from build123d import *

# Parameters (mm, degrees)
BOSS_EXTRU_1_DEPTH      = 50
ESQUISSE2_R             = 8
ENL_V_MAT_EXTRU_1_DEPTH = 42.5
BOSS_EXTRU_3_DEPTH      = 2
BOSS_EXTRU_4_DEPTH      = 8
BOSS_EXTRU_5_DEPTH      = 8.222835
ESQUISSE8_R             = 1.65
ESQUISSE8_R_2           = 3
BOSS_EXTRU_6_DEPTH      = 6.507031
ESQUISSE9_R             = 10.5
ENL_V_MAT_EXTRU_2_DEPTH = 5.007031


with BuildPart() as part:
    # Esquisse1 → Boss.-Extru.1 (new body)
    with BuildSketch(Plane(origin=(0, 0, 0), x_dir=(1, 0, 0), z_dir=(0, 1, 0))):
        with BuildLine():
            ThreePointArc((-34.715340416, 22.739726027), (-41.5, 0), (-34.715340416, -22.739726027))
            ThreePointArc((-34.715340416, -22.739726027), (-31.254191835, -23.461148581), (-30.532769282, -20))
            ThreePointArc((-30.532769282, -20), (-36.5, 0), (-30.532769282, 20))
            ThreePointArc((-30.532769282, 20), (-31.254191835, 23.461148581), (-34.715340416, 22.739726027))
        make_face()
    extrude(amount=BOSS_EXTRU_1_DEPTH)

    # Esquisse2 → Enlèv. mat.-Extru.1 (cut, through all)
    with BuildSketch(Plane(origin=(0, 0, 0), x_dir=(0, 0, -1), z_dir=(1, 0, 0))):
        with Locations((0, 35)):
            Circle(ESQUISSE2_R)
    extrude(amount=-ENL_V_MAT_EXTRU_1_DEPTH, mode=Mode.SUBTRACT)



with BuildPart() as body_2:
    # Esquisse4 → Boss.-Extru.3 (new body)
    with BuildSketch(Plane.ZY.offset(56.5)):
        with BuildLine():
            Line((-2.6, 35), (-2.6, 45))
            Line((-2.6, 45), (-10, 45))
            Line((-10, 45), (-10, 25))
            Line((-10, 25), (10, 25))
            Line((10, 25), (10, 45))
            Line((10, 45), (2.6, 45))
            Line((2.6, 45), (2.6, 35))
            ThreePointArc((2.6, 35), (0, 32.4), (-2.6, 35))
        make_face()
    extrude(amount=BOSS_EXTRU_3_DEPTH)

    # Esquisse6 → Boss.-Extru.4 (add)
    with BuildSketch(Plane.ZY.offset(56.5)):
        Polygon((6.05, 31.507030871), (0, 28.014061743), (-6.05, 31.507030871), (-10, 31.507030871), (-10, 25), (10, 25), (10, 31.507030871), align=None)
    extrude(amount=-BOSS_EXTRU_4_DEPTH)


with BuildPart() as part_1:
    add(part.part)

    add(body_2.part)  # Boss.-Extru.5 merges body 2
    # Esquisse7 → Boss.-Extru.5 (add)
    with BuildSketch(Plane(origin=(-48.5, 0, 0), x_dir=(0, 0, -1), z_dir=(1, 0, 0))):
        with BuildLine():
            Line((10, 31.507030871), (7.197163793, 31.507030871))
            ThreePointArc((7.197163793, 31.507030871), (0, 27), (-7.197163793, 31.507030871))
            Line((-7.197163793, 31.507030871), (-10, 31.507030871))
            Line((-10, 31.507030871), (-10, 25))
            Line((-10, 25), (10, 25))
            Line((10, 25), (10, 31.507030871))
        make_face()
    extrude(amount=BOSS_EXTRU_5_DEPTH)

    # Esquisse8 → Boss.-Extru.6 (add)
    with BuildSketch(Plane.XZ.offset(-25)):
        with BuildLine():
            Line((-54.388582373, 10), (-44.388582373, 10))
            add(Edge.make_bspline(
                [(-82.50013532, 49), (-49.000452969, 40.897437534), (-44.388582373, 10)],
                knots=[0, 0, 0, 1, 1, 1], degree=2))
            ThreePointArc((-82.50013532, 49), (-107.50013532, 44), (-82.50013532, 39))
            add(Edge.make_bspline(
                [(-82.50013532, 39), (-57.708994437, 32.301835207), (-54.388582373, 10)],
                knots=[0, 0, 0, 1, 1, 1], degree=2))
        make_face()
        with Locations((-87.50013532, 44)):
            Circle(ESQUISSE8_R, mode=Mode.SUBTRACT)
        with Locations((-94.50013532, 37)):
            Circle(ESQUISSE8_R, mode=Mode.SUBTRACT)
        with Locations((-101.50013532, 44)):
            Circle(ESQUISSE8_R, mode=Mode.SUBTRACT)
        with Locations((-94.50013532, 51)):
            Circle(ESQUISSE8_R, mode=Mode.SUBTRACT)
        with Locations((-94.50013532, 44)):
            Circle(ESQUISSE8_R_2, mode=Mode.SUBTRACT)
    extrude(amount=-BOSS_EXTRU_6_DEPTH)

    # Esquisse9 → Enlèv. mat.-Extru.2 (cut)
    with BuildSketch(Plane.XZ.offset(-25)):
        with Locations((-94.50013532, 44)):
            Circle(ESQUISSE9_R)
    extrude(amount=-ENL_V_MAT_EXTRU_2_DEPTH, mode=Mode.SUBTRACT)


solid = part_1.part
Geometry check sheet. Reference: the model listing, model coordinates, mm. A direction names the side the tool comes from. Give positions to 0.01 mm unless a question says otherwise; leave off trailing zeros. Order: outer loops, then holes, each group sorted by start corner. A loop starts at its lowest first (then second) coordinate and runs counter-clockwise, first axis right, second up. Notation, with made-up numbers: (84.25, 85) - (100.25, 85) arc R30 ccw to (100.25, 118) - close; hole circle Ø6 at (29, 34.25). An arc over 180 degrees is marked (long way). Answer as a JSON object with one key per item and string values.
(1) Cross-section at B-B (z = 51). Record the cut outline in (x, y), then the cut area to 3 significant figures.
Report:
{"outline": "(-105.45, 25) - (-102.33, 25) - (-102.33, 30.01) - (-96.15, 30.01) - (-96.15, 31.51) - (-105.45, 31.51) - close; (-92.85, 30.01) - (-86.67, 30.01) - (-86.67, 25) - (-83.55, 25) - (-83.55, 31.51) - (-92.85, 31.51) - close", "area": "59.2 mm^2"}
(2) Cross-section at C-C (x = -43). Record the cut outline in (y, z), then the cut area to 3 significant figures.
Report:
{"outline": "(25, -10) - (31.51, -10) - (31.51, -7.2) arc R8 cw to (31.51, 7.2) - (31.51, 10) - (25, 10) - close", "area": "83.7 mm^2"}
(3) Material ranges on line 1 (Y direction, x = -39.6, z = 0); line 2 (Z direction, x = -94.5, y = 28.5); line 3 (Y direction, x = -49.5, z = 9), recorded low to high.
Report:
{"line 1": "0 to 27, 43 to 50", "line 2": "31 to 33.5, 54.5 to 57", "line 3": "25 to 31.51"}
(4) Cross-section at A-A (y = 40). Record the cut outline in (x, z) (3 decimals).
Report:
{"outline": "(-58.5, -10) - (-56.5, -10) - (-56.5, -2.6) - (-58.5, -2.6) - close; (-58.5, 2.6) - (-56.5, 2.6) - (-56.5, 10) - (-58.5, 10) - close; (-41.027, -6.245) arc R41.5 ccw to (-34.715, -22.74) arc R2.5 ccw to (-30.533, -20) arc R36.5 cw to (-35.962, -6.245) - close; (-41.027, 6.245) - (-35.962, 6.245) arc R36.5 cw to (-30.533, 20) arc R2.5 ccw to (-34.715, 22.74) arc R41.5 ccw to start"}
(5) Cross-section at D-D (z = -9). Record the cut outline in (x, y).
Report:
{"outline": "(-58.5, 25) - (-40.51, 25) - (-40.51, 0) - (-35.37, 0) - (-35.37, 50) - (-40.51, 50) - (-40.51, 31.51) - (-56.5, 31.51) - (-56.5, 45) - (-58.5, 45) - close"}
(6) Depth check by flat-ended pin: pin 1 Ø3.5 at (y, z) = (29.5, -0.5) entering from +X; pin 2 Ø3 at (x, z) = (-46.5, 8.5) entering from +Y; pin 3 Ø10 at (y, z) = (39, 0) entering from -X. Enter the tip coordinate at first touch or a pass-through.
Report:
{"pin 1": "x = -48.5", "pin 2": "y = 31.51", "pin 3": "x = -58.5"}
(7) Draft check along Z on faces 1 (the flat face through (-52, 30, -10)), 2 (the flat face through (-37, 50, 0)), 3 (the flat face through (-92, 30.007, 42)). Enter one of: released by +Z, released by -Z, zero draft, split by the parting line, or undercut.
Report:
{"face 1": "released by -Z", "face 2": "zero draft", "face 3": "undercut"}
(8) Tool access check on faces 4 (the flat face through (-57, 45, -6)), 5 (the flat face through (-58.5, 33, -2)), 6 (the flat face through (-52.556, 29.785, 3.067)), 7 (the flat face through (-42, 28, 10)). Record the directions out of +Z, -Z, +X, -X, +Y, -Y that give a thin tool (end or side, any length) a straight path to the whole face; none if there is none.
Report:
{"face 4": "+Z, -Z, -X, +Y", "face 5": "-Z, -X, +Y, -Y", "face 6": "+X, +Y", "face 7": "+Z, +Y, -Y"}
